Work out the finished part from the listing and answer in its coordinate system (mm). A direction names the side the tool comes from. Coordinates: 2 decimals unless noted, no trailing zeros. Order: outer loops, then holes, each group sorted by start corner. A loop starts at its lowest first (then second) coordinate and runs counter-clockwise, first axis right, second up. Notation, with made-up numbers: (33.5, -10) - (56.5, -10) arc R14 cw to (56.5, 14) - close; hole circle Ø8 at (67.25, -36). An arc over 180 degrees is marked (long way). Answer as a JSON object with one key per item and string values. Group by question number.
1) Section C-C (z = 8.25) is taken. Count the separate pieces of the cut face and the enclosed holes in it, plus the area to 3 significant figures.
2) Find the intervals of material crossed by line 1 along X through (y, z) = (-111, 9.75); line 2 along X through (y, z) = (-90, 5.75); line 3 along Y through (x, z) = (55.5, 6.25), in increasing order.
3) Section A-A (x = 53) is taken. Give the vertices of the cut face in (y, z), plus the area to 3 significant figures.
4) Section B-B (y = -205) is taken. Give the vertices of the cut face in (x, z), plus the area to 3 significant figures.
5) The mould has two halves that part along Y. Classify faces 4 (the face through (24, 10, 7)), 5 (the face through (13, -3.4, 7)), 6 (the face through (105, -172, 0)), 7 (the face through (101, -232, 7)): released by +Y, released by -Y, zero draft, split by the parting line, or undercut.
6) A tool of negligible diameter and unlimited length cuts with its end or side. For faces 1 (the face through (3.4, -180, 7)), 2 (the face through (54, -230, 0)), 3 (the face through (9, 0, 7)), from which of +Z, -Z, +X, -X, +Y, -Y can it reach the whole face along a straight path? Write none if from no direction.
7) Each of these flat-tipped pins is pushed along its axis until it touches: P1, Ø1, axis at x = 34.5, z = 9.5, coming from the -Y side; P2, Ø4.5, axis at x = 56.5, z = 10, coming from the +Y side. Where does it stop, or does it pass through?
from build123d import *

# Parameters (mm, degrees)
F0_R        = 1.75
F1_DEPTH    = 15
F2_T        = 3.4
F2_T3_DEPTH = 21.8
F3_R        = 2
F5_DEPTH    = 200


# Not quite as in the source:
# - a shell that OpenCascade refuses in one call is made with other operations: the cavity is built on its own and cut out


with BuildPart() as f1:
    # F0 (on Top) → F1 (new body)
    with BuildSketch(Plane.XY):
        Polygon((17, 0), (0, 0), (0, -232), (15.75, -232), (10.75, -221.25), (37.25, -221.25), (32.25, -232), (75.55, -232), (70.55, -221.25), (97.05, -221.25), (92.05, -232), (107.8, -232), (107.8, 0), (90.8, 0), (95.8, 10), (71.8, 10), (76.8, 0), (31, 0), (36, 10), (12, 10), align=None)
        with Locations((5.9, -227)):
            Circle(F0_R, mode=Mode.SUBTRACT)
        with Locations((5.9, -191.5)):
            Circle(F0_R, mode=Mode.SUBTRACT)
        with Locations((5.9, -169)):
            Circle(F0_R, mode=Mode.SUBTRACT)
        with Locations((5.9, -133.5)):
            Circle(F0_R, mode=Mode.SUBTRACT)
        with Locations((101.9, -227)):
            Circle(F0_R, mode=Mode.SUBTRACT)
        with Locations((101.9, -191.5)):
            Circle(F0_R, mode=Mode.SUBTRACT)
        with Locations((101.9, -169)):
            Circle(F0_R, mode=Mode.SUBTRACT)
        with Locations((101.9, -133.5)):
            Circle(F0_R, mode=Mode.SUBTRACT)
        with Locations((5.9, -111)):
            Circle(F0_R, mode=Mode.SUBTRACT)
        with Locations((5.9, -75.5)):
            Circle(F0_R, mode=Mode.SUBTRACT)
        with Locations((5.9, -53)):
            Circle(F0_R, mode=Mode.SUBTRACT)
        with Locations((5.9, -17.5)):
            Circle(F0_R, mode=Mode.SUBTRACT)
        with Locations((101.9, -111)):
            Circle(F0_R, mode=Mode.SUBTRACT)
        with Locations((101.9, -75.5)):
            Circle(F0_R, mode=Mode.SUBTRACT)
        with Locations((101.9, -53)):
            Circle(F0_R, mode=Mode.SUBTRACT)
        with Locations((101.9, -17.5)):
            Circle(F0_R, mode=Mode.SUBTRACT)
    extrude(amount=F1_DEPTH)

    # F2: shell of thickness 3.4, made by hand


with BuildPart() as f2_core1:
    # F2_t2: copy of F1
    add(f1.part)

    # the walls: a layer under each face that stays
    f2_faces = [f2_core1.faces().sort_by_distance(p)[0] for p in [
        (8.5, 0, 7.5),
        (0, -116, 7.5),
        (7.875, -232, 7.5),
        (13.25, -226.625, 7.5),
        (24, -221.25, 7.5),
        (34.75, -226.625, 7.5),
        (53.9, -232, 7.5),
        (73.05, -226.625, 7.5),
        (83.8, -221.25, 7.5),
        (94.55, -226.625, 7.5),
        (99.925, -232, 7.5),
        (107.8, -116, 7.5),
        (99.3, 0, 7.5),
        (93.3, 5, 7.5),
        (83.8, 10, 7.5),
        (74.3, 5, 7.5),
        (53.9, 0, 7.5),
        (33.5, 5, 7.5),
        (24, 10, 7.5),
        (14.5, 5, 7.5),
        (4.15, -227, 7.5),
        (4.15, -191.5, 7.5),
        (4.15, -169, 7.5),
        (4.15, -133.5, 7.5),
        (100.15, -227, 7.5),
        (100.15, -191.5, 7.5),
        (100.15, -169, 7.5),
        (100.15, -133.5, 7.5),
        (4.15, -111, 7.5),
        (4.15, -75.5, 7.5),
        (4.15, -53, 7.5),
        (4.15, -17.5, 7.5),
        (100.15, -111, 7.5),
        (100.15, -75.5, 7.5),
        (100.15, -53, 7.5),
        (100.15, -17.5, 7.5),
    ]]
    thicken(f2_faces, amount=-F2_T, mode=Mode.SUBTRACT)

    # F2_s4 → F2_t3 (cut)
    with BuildSketch(Plane.XY.offset(-3.4)):
        Polygon((16.9695894755, 0.0187947378), (17, -3.4), (22.5013155617, -3.4), (20.0410524494, 1.5205262247), align=None)
        Polygon((10.7808285178, -221.2696611545), (7.6671482196, -222.683884549), (5.4188298247, -217.85), (10.75, -217.85), align=None)
        Polygon((37.2191714822, -221.2696611545), (37.25, -217.85), (42.5811701753, -217.85), (40.3328517804, -222.683884549), align=None)
        Polygon((70.5808285178, -221.2696611545), (67.4671482196, -222.683884549), (65.2188298247, -217.85), (70.55, -217.85), align=None)
        Polygon((97.0191714822, -221.2696611545), (97.05, -217.85), (102.3811701753, -217.85), (100.1328517804, -222.683884549), align=None)
        Polygon((90.8304105245, 0.0187947378), (90.8, -3.4), (85.2986844383, -3.4), (87.7589475506, 1.5205262247), align=None)
        Polygon((76.7695894755, 0.0187947378), (79.8410524494, 1.5205262247), (82.3013155617, -3.4), (76.8, -3.4), align=None)
        Polygon((31.0304105245, 0.0187947378), (31, -3.4), (25.4986844383, -3.4), (27.9589475506, 1.5205262247), align=None)
    extrude(amount=F2_T3_DEPTH, mode=Mode.SUBTRACT)


with BuildPart() as f1_1:
    add(f1.part)

    # what is left inside the walls is the cavity
    f2_cavity = [f2_core1.part.solids().sort_by_distance(p)[0] for p in [
        (53.9, -150.2, 14.966),
    ]]
    add(f2_cavity, mode=Mode.SUBTRACT)

    # F3
    f3_edges = [f1_1.edges().sort_by_distance(p)[0] for p in [
        (15.75, -232, 7.5),
        (32.25, -232, 7.5),
        (75.55, -232, 7.5),
        (92.05, -232, 7.5),
        (12, 10, 7.5),
        (36, 10, 7.5),
        (71.8, 10, 7.5),
        (95.8, 10, 7.5),
    ]]
    fillet(f3_edges, radius=F3_R)

    # F4 (on face) → F5 (cut)
    with BuildSketch(Plane.YZ.offset(107.8)):
        with BuildLine():
            Line((-210.2734148502, 0), (-193.2988762856, 0))
            ThreePointArc((-193.2988762856, 0), (-201.7861455679, 5.2826077701), (-210.2734148502, 0))
        make_face()
        with BuildLine():
            ThreePointArc((-135.2988762856, 0), (-143.7861455679, 5.2826077701), (-152.2734148502, 0))
            Line((-152.2734148502, 0), (-135.2988762856, 0))
        make_face()
        with BuildLine():
            ThreePointArc((-77.2988762856, 0), (-85.7861455679, 5.2826077701), (-94.2734148502, 0))
            Line((-94.2734148502, 0), (-77.2988762856, 0))
        make_face()
        with BuildLine():
            ThreePointArc((-19.2988762856, 0), (-27.7861455679, 5.2826077701), (-36.2734148502, 0))
            Line((-36.2734148502, 0), (-19.2988762856, 0))
        make_face()
    extrude(amount=-F5_DEPTH, mode=Mode.SUBTRACT)


solid = f1_1.part
Report:
{
 "1": {"separate pieces": "1", "enclosed holes": "17", "area": "3,540 mm²"},
 "2": {"line 1": "x = 0 to 4.15, 7.65 to 11.05, 96.75 to 100.15, 103.65 to 107.8", "line 2": "x = 0 to 3.4, 104.4 to 107.8", "line 3": "y = -232 to -228.6, -3.4 to 0"},
 "3": {"outline": "(-232, 0) - (-228.6, 0) - (-228.6, 15) - (-232, 15) - close; (-3.4, 0) - (0, 0) - (0, 15) - (-3.4, 15) - close", "area": "102 mm²"},
 "4": {"outline": "(0, 4.72) - (3.4, 4.72) - (3.4, 15) - (0, 15) - close; (104.4, 4.72) - (107.8, 4.72) - (107.8, 15) - (104.4, 15) - close", "area": "69.9 mm²"},
 "5": {"face 4": "released by +Y", "face 5": "undercut", "face 6": "zero draft", "face 7": "released by -Y"},
 "6": {"face 1": "+Z, -Z", "face 2": "-Z, +X, -X, +Y, -Y", "face 3": "+Z, -Z, -X"},
 "7": {"P1": "stops at y = -231.96", "P2": "stops at y = 0"}
}
